Work out the finished part from the listing and answer in its coordinate system (mm). A direction names the side the tool comes from. Coordinates: 2 decimals unless noted, no trailing zeros. Order: outer loops, then holes, each group sorted by start corner. A loop starts at its lowest first (then second) coordinate and runs counter-clockwise, first axis right, second up.
1. The part is cut by section A-A, the plane z = 5.25. Give the vertices of the cut face in (x, y), then the cut area to 3 significant figures.
2. The part is cut by section D-D, the plane z = 22. Give the vertices of the cut face in (x, y).
3. A tool of negligible diameter and unlimited length cuts with its end or side. For faces 3 (the flat face through (27, 21, 14.5)), 4 (the cylindrical face through (20.302, 0.088, 0.493)), 5 (the flat face through (-17.9, 0, 26)), 6 (the flat face through (6, -29.25, 12)), from which of +Z, -Z, +X, -X, +Y, -Y can it reach the whole face along a straight path? Write none if from no direction.
4. Flat-ended cylindrical pins translate along their axes: pin 1 Ø1.8 at (y, z) = (2, 26) entering from -X; pin 2 Ø5 at (x, y) = (17, -26) entering from +Z; pin 3 Ø2 at (x, z) = (-13, 23.5) entering from -Y. Find the tip coordinate at first contact, or state that the pin passes through.
5. The part is cut by section B-B, the plane x = 22.3. Give the vertices of the cut face in (y, z), then the cut area to 3 significant figures.
6. Determine the mould class of faces 1 (the cylindrical face through (-23.9, -0.2, 21.2)), 2 (the cylindrical face through (25.334, 30.264, 20.794)) for opening direction Y: +Y half, -Y half, draft (parallel to the pull), parting line (faces both ways), or undercut.
7. Find the intervals of material crossed by probe 1 along X at (y, z) = (0, 0.25); probe 2 along X at (y, z) = (-27, 11.5); probe 3 along Y at (x, z) = (-24.5, 21), in increasing order.
8. The part is cut by section C-C, the plane x = -15.5. Give the vertices of the cut face in (y, z), then the cut area to 4 significant figures.
```python
from build123d import *

# Parameters (mm, degrees)
F0_W      = 55.8
F0_H      = 62.5
F0_R      = 2
F0_R_2    = 1.5
F1_DEPTH  = 1
F3_DEPTH  = 2
F5_W      = 58.5
F5_H      = 13.5
F6_DEPTH  = 1.5
F10_DEPTH = 1
F14_DEPTH = 26.4
F16_W     = 3
F16_H     = 0.7499982331
F17_DEPTH = 1
F18_R     = 0.7
F19_DEPTH = 15


with BuildPart() as f1:
    # F0 (on Top) → F1 (new body)
    with BuildSketch(Plane.XY):
        Rectangle(F0_W, F0_H)
        with Locations((-22.3, 0)):
            Circle(F0_R, mode=Mode.SUBTRACT)
        Circle(F0_R_2, mode=Mode.SUBTRACT)
        with Locations((22.3, 0)):
            Circle(F0_R, mode=Mode.SUBTRACT)
    extrude(amount=F1_DEPTH)

    # F4: F3 across plane


with BuildPart() as f3:
    # F2 (on face) → F3 (new body)
    with BuildSketch(Plane.XZ.offset(31.25)):
        with BuildLine():
            Line((-27.9, 14.5), (-27.9, 1))
            Line((-27.9, 1), (27.9, 1))
            Line((27.9, 1), (27.9, 14.5))
            ThreePointArc((27.9, 14.5), (25.2639610307, 20.8639610307), (18.9, 23.5))
            Line((18.9, 23.5), (-18.9, 23.5))
            ThreePointArc((-18.9, 23.5), (-25.2639610307, 20.8639610307), (-27.9, 14.5))
        make_face()
    extrude(amount=-F3_DEPTH)


with BuildPart() as f1_1:
    add(f1.part)
    add(f3.part.mirror(Plane.XZ))


    add(f3.part)  # F6 merges F3
    # F5 (on face) → F6 (join)
    with BuildSketch(Plane.YZ.offset(27.9)):
        with Locations((0, 7.75)):
            Rectangle(F5_W, F5_H)
    extrude(amount=-F6_DEPTH)

    # F7: F1 across plane


with BuildPart() as f1_2:
    add(f1_1.part)
    add(f1_1.part.mirror(Plane.YZ))

    # F9 (on offset) → F10 (join)
    with BuildSketch(Plane.YZ.offset(0.5)):
        Polygon((-18.05, 8.8), (-29.25, 20), (-29.25, 0), (-4, 0), (-4, 8.8), align=None)
    extrude(amount=-F10_DEPTH)

    # F11: F1 across plane


with BuildPart() as f1_3:
    add(f1_2.part)
    add(f1_2.part.mirror(Plane.XZ))

    # F13 (on offset) → F14 (join)
    with BuildSketch(Plane.XZ.offset(13.2)):
        with BuildLine():
            Line((-17.9, 25.599895397), (-17.9, 27.204427321))
            ThreePointArc((-17.9, 27.204427321), (-24.8888113544, 22.4176611255), (-27.9, 14.5))
            Line((-27.9, 14.5), (-26.3714103808, 14.5))
            ThreePointArc((-26.3714103808, 14.5), (-23.805942074, 21.3246680061), (-17.9, 25.599895397))
        make_face()
    extrude(amount=-F14_DEPTH)

    # F15: F1 across plane


with BuildPart() as f1_4:
    add(f1_3.part)
    add(f1_3.part.mirror(Plane.YZ))

    # F16 (on face) → F17 (cut)
    with BuildSketch(Plane.XY.offset(1)):
        with Locations((-6.5461898372, 23.3516955865)):
            Rectangle(F16_W, F16_H)
        Polygon((7.3961903043, 22.9248698354), (8.5211903043, 22.9248698354), (8.5211903043, 23.6748680685), (7.3961903043, 23.6748680685), (7.3961903043, 24.7998698354), (6.6461903043, 24.7998698354), (6.6461903043, 23.6748680685), (5.5211903043, 23.6748680685), (5.5211903043, 22.9248698354), (6.6461903043, 22.9248698354), (6.6461903043, 21.7998698354), (7.3961903043, 21.7998698354), align=None)
        with Locations((6.5461898372, -23.3516955865)):
            Rectangle(F16_W, F16_H)
        Polygon((-6.1711898372, -23.7266947031), (-5.0461898372, -23.7266947031), (-5.0461898372, -22.97669647), (-6.1711898372, -22.97669647), (-6.1711898372, -21.8516947031), (-6.9211898372, -21.8516947031), (-6.9211898372, -22.97669647), (-8.0461898372, -22.97669647), (-8.0461898372, -23.7266947031), (-6.9211898372, -23.7266947031), (-6.9211898372, -24.8516947031), (-6.1711898372, -24.8516947031), align=None)
    extrude(amount=-F17_DEPTH, mode=Mode.SUBTRACT)

    # F18 (on face) → F19 (join)
    with BuildSketch(Plane.XZ.offset(31.25)):
        with Locations((-1.4, 2.7)):
            Circle(F18_R)
        with Locations((1.4, 2.7)):
            Circle(F18_R)
    extrude(amount=F19_DEPTH)


solid = f1_4.part
```
Geometry says:
1. outline: (-27.9, -31.25) - (27.9, -31.25) - (27.9, 31.25) - (-27.9, 31.25) - close; hole (-26.4, -29.25) - (-0.5, -29.25) - (-0.5, -4) - (0.5, -4) - (0.5, -29.25) - (26.4, -29.25) - (26.4, 29.25) - (0.5, 29.25) - (0.5, 4) - (-0.5, 4) - (-0.5, 29.25) - (-26.4, 29.25) - close
1. area: 449 mm2
2. outline: (-25.21, -13.2) - (-23.25, -13.2) - (-23.25, 13.2) - (-25.21, 13.2) - close; (-23.87, -31.25) - (23.87, -31.25) - (23.87, -29.25) - (-23.87, -29.25) - close; (-23.87, 29.25) - (23.87, 29.25) - (23.87, 31.25) - (-23.87, 31.25) - close; (23.25, -13.2) - (25.21, -13.2) - (25.21, 13.2) - (23.25, 13.2) - close
3. face 3: +Z, +X
3. face 4: -Z
3. face 5: +Z, +Y, -Y
3. face 6: +Z
4. pin 1: stops at x = -22.11
4. pin 2: stops at z = 1
4. pin 3: stops at y = -31.25
5. outline: (-31.25, 0) - (-2, 0) - (-2, 1) - (-29.25, 1) - (-29.25, 22.83) - (-31.25, 22.83) - close; (-13.2, 22.97) - (13.2, 22.97) - (13.2, 24.96) - (-13.2, 24.96) - close; (2, 0) - (31.25, 0) - (31.25, 22.83) - (29.25, 22.83) - (29.25, 1) - (2, 1) - close
5. area: 198 mm2
6. face 1: undercut
6. face 2: draft
7. probe 1: x = -27.9 to -24.3, -20.3 to -1.5, 1.5 to 20.3, 24.3 to 27.9
7. probe 2: x = -27.9 to -26.4, -0.5 to 0.5, 26.4 to 27.9
7. probe 3: y = -31.25 to -29.25, -13.2 to 13.2, 29.25 to 31.25
8. outline: (-31.25, 0) - (31.25, 0) - (31.25, 23.5) - (29.25, 23.5) - (29.25, 1) - (-29.25, 1) - (-29.25, 23.5) - (-31.25, 23.5) - close
8. area: 152.5 mm2
